Geometry: final body of the model. Coordinates: model frame, mm. A direction names the side the tool comes from. Give positions to 0.01 mm unless a question says otherwise; leave off trailing zeros. Write each loop counter-clockwise with the first axis right and the second up, starting at its lowest first coordinate (ties: lowest second). Pieces come first, ordered by that corner, then holes. Notation, with made-up numbers: M 35.5,77.25 L 69.5,77.25 A14 ccw 69.5,84.25 Z; hole C 20.5,33.25 d8. An arc over 180 degrees is marked long. One line per question, with ' | ' between items.
from build123d import *

# Parameters (mm, degrees)
SKETCH_R             = 20
PAD_DEPTH            = 7
SKETCH001_R          = 3
PAD001_DEPTH         = 5
SKETCH002_R          = 20
SKETCH002_R_2        = 19
PAD002_DEPTH         = 7.6
SKETCH003_W          = 53
SKETCH003_H          = 60
PAD003_DEPTH         = 3.5
SKETCH004_W          = 53
SKETCH004_H          = 60
SKETCH004_W_2        = 51
SKETCH004_H_2        = 58
PAD004_DEPTH         = 15
SKETCH006_R          = 3
POCKET_DEPTH         = 3
SKETCH005_R          = 5
POCKET001_DEPTH      = 3.501
POCKET001_DEPTH_BACK = -15.001


with BuildPart() as part:
    # Sketch → Pad (new body)
    with BuildSketch(Plane.XY):
        Circle(SKETCH_R)
    extrude(amount=PAD_DEPTH)

    # Sketch001 → Pad001 (join)
    with BuildSketch(Plane.XY):
        with BuildLine():
            add(Edge.make_bspline(
                [(-14.633789, 13.632763), (-10.829835, 26.268087), (0, 32.822822), (10.829835, 26.268087), (14.633789, 13.632763)],
                knots=[0, 0, 0, 0, 0.5, 1, 1, 1, 1], degree=3))
            Line((14.633789, 13.632763), (-14.633789, 13.632763))
        make_face()
        with Locations((0, 24.48224)):
            Circle(SKETCH001_R, mode=Mode.SUBTRACT)
    extrude(amount=PAD001_DEPTH)

    # Sketch002 → Pad002 (join)
    with BuildSketch(Plane.XY):
        Circle(SKETCH002_R)
        Circle(SKETCH002_R_2, mode=Mode.SUBTRACT)
    extrude(amount=PAD002_DEPTH)

    # Sketch003 → Pad003 (join)
    with BuildSketch(Plane.XY):
        with Locations((0, 5)):
            Rectangle(SKETCH003_W, SKETCH003_H)
    extrude(amount=-PAD003_DEPTH)

    # Sketch004 → Pad004 (join)
    with BuildSketch(Plane.XY):
        with Locations((0, 5)):
            Rectangle(SKETCH004_W, SKETCH004_H)
        with Locations((0, 5)):
            Rectangle(SKETCH004_W_2, SKETCH004_H_2, mode=Mode.SUBTRACT)
    extrude(amount=PAD004_DEPTH)

    # Sketch006 → Pocket (cut)
    with BuildSketch(Plane.XY):
        with Locations((0, 24.48224)):
            Circle(SKETCH006_R)
    extrude(amount=-POCKET_DEPTH, mode=Mode.SUBTRACT)

    # Sketch005 → Pocket001 (cut, two sides)
    with BuildSketch(Plane.XY) as pocket001_sk:
        Circle(SKETCH005_R)
    extrude(amount=-POCKET001_DEPTH, mode=Mode.SUBTRACT)
    extrude(pocket001_sk.sketch, amount=-POCKET001_DEPTH_BACK, mode=Mode.SUBTRACT)


solid = part.part
(1) Cut plane B-B, the plane z = 11.75. Return loops of the section in (x, y).
Working result:
outline: M -26.5,-25 L 26.5,-25 L 26.5,35 L -26.5,35 Z; hole M -25.5,-24 L 25.5,-24 L 25.5,34 L -25.5,34 Z
(2) Cut plane D-D, the plane z = 2.75. Count the separate pieces of the cut face and the enclosed holes in it, then the cut area to 3 significant figures.
Working result:
separate pieces: 2 | enclosed holes: 3 | area: 1,580 mm^2
(3) Draft query along Y for faces 3 (the face through (0, 35, 6)), 4 (the face through (-0.4, 5.4, -3.5)), 5 (the face through (0, -25, 6)), 6 (the face through (17, 12, 0)). Return one class per face: released by +Y, released by -Y, zero draft, split by the parting line, or undercut.
Working result:
face 3: released by +Y | face 4: zero draft | face 5: released by -Y | face 6: undercut
(4) Cut plane C-C, the plane x = 21. Return loops of the section in (y, z).
Working result:
outline: M -25,-3.5 L 35,-3.5 L 35,15 L 34,15 L 34,0 L -24,0 L -24,15 L -25,15 Z
(5) First-contact query: P1, Ø11.5, axis at x = -5.5, y = 4.5, coming from the +Z side; P2, Ø6, axis at x = 0, y = 0, coming from the -Z side; P3, Ø10, axis at x = -13.5, y = 22.5, coming from the +Z side; P4, Ø5, axis at x = 0, y = 24.48, coming from the +Z side. Flat tips, straight axial feed; report the tip coordinate or a pass-through.
Working result:
P1: stops at z = 7 | P2: passes through | P3: stops at z = 5 | P4: stops at z = -3
(6) Cut plane A-A, the plane y = 0. Return loops of the section in (x, z).
Working result:
outline: M -26.5,-3.5 L -5,-3.5 L -5,7 L -19,7 L -19,7.6 L -20,7.6 L -20,0 L -25.5,0 L -25.5,15 L -26.5,15 Z; M 5,-3.5 L 26.5,-3.5 L 26.5,15 L 25.5,15 L 25.5,0 L 20,0 L 20,7.6 L 19,7.6 L 19,7 L 5,7 Z
(7) Set-up query: faces 1 (the face through (4, -4, 7)), 2 (the face through (-1.08, -4.88, 1.82)). Return all of +Z, -Z, +X, -X, +Y, -Y with unobstructed straight access to the full face (end or side cutting, diameter ignored); none if empty.
Working result:
face 1: +Z | face 2: +Z, -Z
(8) Material intervals for L1, parallel to Y at x = 0, z = 0.25; L2, parallel to X at y = 0, z = 2.5; L3, parallel to Y at x = 0.5, z = 10.75, sorted ascending. Write a range as [from, to].
Working result:
L1: y = [-25, -24], [-20, -5], [5, 21.48], [27.48, 29.55], [34, 35] | L2: x = [-26.5, -25.5], [-20, -5], [5, 20], [25.5, 26.5] | L3: y = [-25, -24], [34, 35]
